Source: three-view drawing plus pictorial views. Frame: mm from the lowest corner of the part. A direction names the side the tool comes from. Round coordinates to 2 decimals unless told otherwise and drop trailing zeros. Order: outer loops, then holes, each group sorted by start corner. A loop starts at its lowest first (then second) coordinate and runs counter-clockwise, first axis right, second up. Notation, with made-up numbers: (60.25, 23) - (93.25, 23) arc R25 ccw to (93.25, 35) - close; hole circle Ø4 at (9, 18). An arc over 180 degrees is marked (long way). One line per item, written item: value. Start each with the question number.
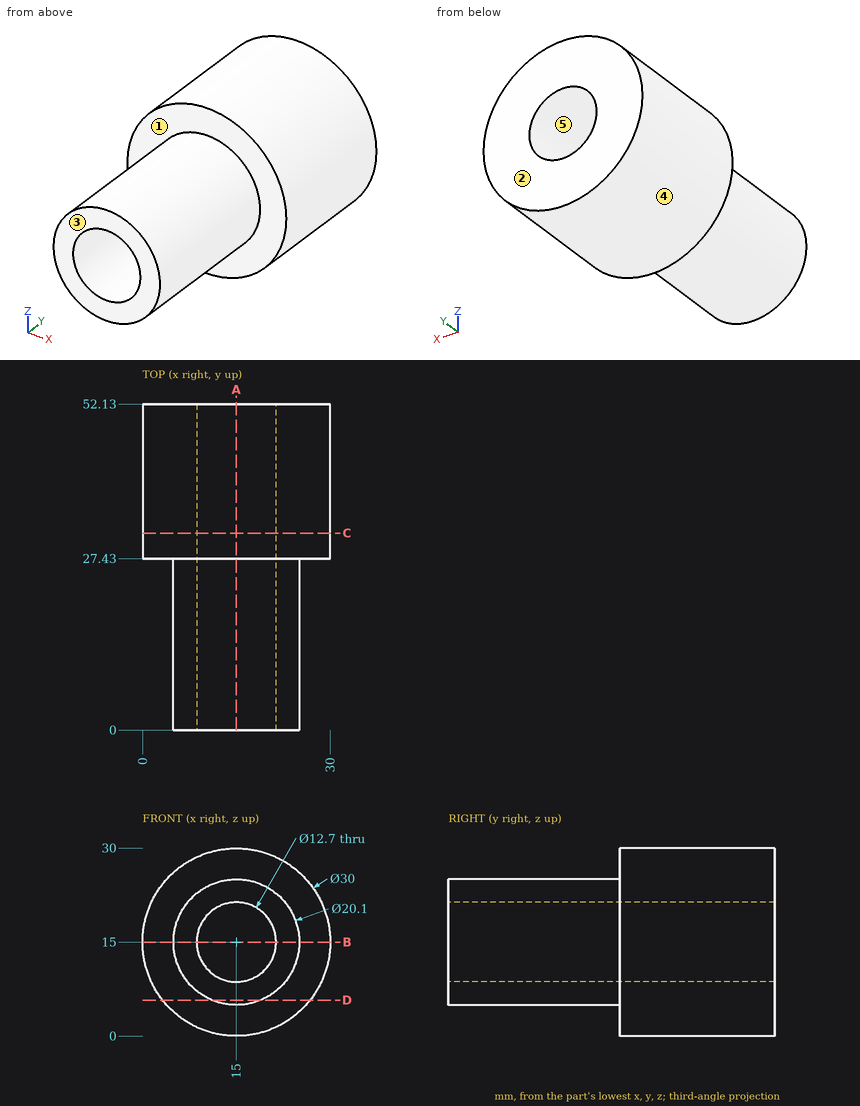
Item 1: First-contact query: pin 1 Ø8 at (y, z) = (36, 7.5) entering from -X; pin 2 Ø11.5 at (x, z) = (15, 15) entering from +Y; pin 3 Ø3 at (y, z) = (26.5, 25) entering from +X; pin 4 Ø2 at (x, y) = (22, 24.5) entering from -Z. Flat tips, straight axial feed; report the tip coordinate or a pass-through.
Item 2: Section query D-D on z = 5.75. Return loops of the section in (x, y).
Item 3: Section query A-A on x = 15. Return loops of the section in (y, z).
Item 4: Section query B-B on z = 15. Return loops of the section in (x, y).
Item 5: Section query C-C on y = 31.5. Return loops of the section in (x, z).
Item 6: Line query: L1, parallel to Z at x = 15, y = 29; L2, parallel to Z at x = 15, y = 21; L3, parallel to X at y = 38.5, z = 16.75. Output: solid intervals per line, ascending.
Item 7: Pull-direction query (X, two-part tool) for the marked faces 3, 4 and 5; classes: released by +X, released by -X, zero draft, split by the parting line, or undercut.
Item 8: Reachability of the marked faces 1 and 2 from +Z, -Z, +X, -X, +Y, -Y: full face, straight path, thin tool, end or side. Return the list, or none.
Geometry results:
1. pin 1: stops at x = 0.41
1. pin 2: passes through
1. pin 3: stops at x = 27.13
1. pin 4: stops at z = 6.94
2. outline: (3.19, 27.43) - (11.07, 27.43) - (11.07, 0) - (18.93, 0) - (18.93, 27.43) - (26.81, 27.43) - (26.81, 52.13) - (3.19, 52.13) - close
3. outline: (0, 4.95) - (27.43, 4.95) - (27.43, 0) - (52.13, 0) - (52.13, 8.65) - (0, 8.65) - close; (0, 21.35) - (52.13, 21.35) - (52.13, 30) - (27.43, 30) - (27.43, 25.05) - (0, 25.05) - close
4. outline: (0, 27.43) - (4.95, 27.43) - (4.95, 0) - (8.65, 0) - (8.65, 52.13) - (0, 52.13) - close; (21.35, 0) - (25.05, 0) - (25.05, 27.43) - (30, 27.43) - (30, 52.13) - (21.35, 52.13) - close
5. outline: circle Ø30 at (15, 15); hole circle Ø12.7 at (15, 15)
6. L1: z = 0 to 8.65, 21.35 to 30
6. L2: z = 4.95 to 8.65, 21.35 to 25.05
6. L3: x = 0.1 to 8.9, 21.1 to 29.9
7. face 3: zero draft
7. face 4: split by the parting line
7. face 5: undercut
8. face 1: -Y
8. face 2: +Z, -Z, +X, -X, +Y
